from build123d import *

# Parameters (mm, degrees)
PAD_DEPTH       = 10
SKETCH001_R     = 17
POCKET_DEPTH    = 8
FILLET_R        = 2
FILLET001_R     = 2
SKETCH002_R     = 3
POCKET001_DEPTH = 5
FILLET002_R     = 2
FILLET003_R     = 2
SKETCH003_R     = 0.5
POCKET002_DEPTH = 5


with BuildPart() as part:
    # Sketch → Pad (new body)
    with BuildSketch(Plane.XY):
        with BuildLine():
            ThreePointArc((29.142732, 7.120476), (26.750427, 13.579935), (22.947847, 19.323465))
            Line((22.947847, 19.323465), (34.497449, 29.048923))
            ThreePointArc((34.497449, 29.048923), (0.205805, 45.098466), (-34.230891, 29.362562))
            Line((-22.770532, 19.532099), (-34.230891, 29.362562))
            ThreePointArc((-22.770532, 19.532099), (-26.452647, 14.151236), (-28.885266, 8.101937))
            Line((-28.885266, 8.101937), (-43.374809, 11.984403))
            ThreePointArc((-43.374809, 11.984403), (-43.973621, 9.556182), (-44.436607, 7.098445))
            Line((-44.436607, 7.098445), (-11.603749, -16.289659))
            ThreePointArc((-11.603749, -16.289659), (0.53379, -19.992875), (12.456435, -15.647276))
            Line((43.994501, 9.459593), (12.456435, -15.647276))
            ThreePointArc((43.994501, 9.459593), (43.401023, 11.889122), (42.673487, 14.281929))
            Line((29.142732, 7.120476), (42.673487, 14.281929))
        make_face()
    extrude(amount=PAD_DEPTH)

    # Sketch001 → Pocket (cut)
    with BuildSketch(Plane.XY.offset(10)):
        Circle(SKETCH001_R)
    extrude(amount=-POCKET_DEPTH, mode=Mode.SUBTRACT)

    # Fillet
    fillet_edges = [part.edges().sort_by_distance(p)[0] for p in [
        (-34.230891, 29.362562, 5),
    ]]
    fillet(fillet_edges, radius=FILLET_R)

    # Fillet001
    fillet001_edges = [part.edges().sort_by_distance(p)[0] for p in [
        (34.497449, 29.048923, 5),
    ]]
    fillet(fillet001_edges, radius=FILLET001_R)

    # Sketch002 → Pocket001 (cut)
    with BuildSketch(Plane.XY.offset(2)):
        Circle(SKETCH002_R)
    extrude(amount=-POCKET001_DEPTH, mode=Mode.SUBTRACT)

    # Fillet002
    fillet002_edges = [part.edges().sort_by_distance(p)[0] for p in [
        (-17, 0, 10),
    ]]
    fillet(fillet002_edges, radius=FILLET002_R)

    # Fillet003
    fillet003_edges = [part.edges().sort_by_distance(p)[0] for p in [
        (0.205805, 45.098466, 10),
    ]]
    fillet(fillet003_edges, radius=FILLET003_R)

    # Sketch003 → Pocket002 (cut)
    with BuildSketch(Plane.XY.offset(2)):
        with Locations((7.5, 3)):
            Circle(SKETCH003_R)
        with Locations((-7.5, -3)):
            Circle(SKETCH003_R)
    extrude(amount=-POCKET002_DEPTH, mode=Mode.SUBTRACT)


solid = part.part
Input: part model. Units: mm. Frame: model coordinates. A direction names the side the tool comes from. Coordinates: 2 decimals unless noted, no trailing zeros. Order: outer loops, then holes, each group sorted by start corner. A loop starts at its lowest first (then second) coordinate and runs counter-clockwise, first axis right, second up. Notation, with made-up numbers: M 28,17.5 L 36,17.5 A27 cw 36,53.5 Z; hole C 0.5,16.5 d2. An arc over 180 degrees is marked long. Answer in a Markdown table with one row per item.
(1) Section query B-B, the plane z = 6. Output: boundary loops of the cut face in (x, y).
Numbers:
| item | result |
|---|---|
| outline | M -44.44,7.1 L -11.6,-16.29 A20 ccw 12.46,-15.65 L 43.99,9.46 A45 ccw 42.67,14.28 L 29.14,7.12 A30 ccw 22.95,19.32 L 32.93,27.73 A2 ccw 33.11,30.62 A45.1 ccw -32.83,30.92 A2 ccw -32.68,28.03 L -22.77,19.53 A30 ccw -28.89,8.1 L -43.37,11.98 A45 ccw Z; hole C 0,0 d34 |
(2) Section query A-A, the plane y = 0. Output: boundary loops of the cut face in (x, z).
Numbers:
| item | result |
|---|---|
| outline | M -34.47,0 L -3,0 L -3,2 L -17,2 L -17,8 A2 ccw -19,10 L -34.47,10 Z; M 3,0 L 32.11,0 L 32.11,10 L 19,10 A2 ccw 17,8 L 17,2 L 3,2 Z |
(3) Material intervals for line 1 (Y direction, x = 0, z = 6.3); line 2 (Z direction, x = 10, y = -8); line 3 (X direction, y = -1.5, z = 4.5), sorted ascending. Write a range as [from, to].
Numbers:
| item | result |
|---|---|
| line 1 | y = [-20, -17], [17, 45.1] |
| line 2 | z = [0, 2] |
| line 3 | x = [-32.37, -16.93], [16.93, 30.23] |
(4) Access query for faces 4 (the flat face through (4, 0, 2)), 5 (the cylindrical face through (27.597, 24.025, 9.43)), 6 (the cylindrical face through (-27.24, 24.16, 9.43)), 7 (the flat face through (27.87, 23.47, 3.94)), 8 (the flat face through (-36.029, 10.016, 4.93)). Directions: +Z, -Z, +X, -X, +Y, -Y. A direction counts if a zero-diameter tool reaches every point of the face in a straight line with its end or side. Return the directions, or none.
Numbers:
| item | result |
|---|---|
| face 4 | +Z |
| face 5 | +Z, +X |
| face 6 | +Z, -X |
| face 7 | +Z, -Z, +X |
| face 8 | +Z, -Z |
(5) Contact query for flat-ended pins moving along their axis: pin 1 Ø1 at (x, z) = (-28, 5) entering from +Y; pin 2 Ø3 at (y, z) = (10, 8) entering from -X; pin 3 Ø6 at (x, z) = (29.5, 3.5) entering from -Y; pin 4 Ø3.5 at (x, y) = (0, 0) entering from +Z. Output: stop coordinate, or through.
Numbers:
| item | result |
|---|---|
| pin 1 | stops at y = 35.74 |
| pin 2 | stops at x = -44.19 |
| pin 3 | stops at y = -4.47 |
| pin 4 | passes through |
(6) Draft query along X for faces 1 (the cylindrical face through (-33.374, 29.465, 4.056)), 2 (the flat face through (35.81, 10.65, 4.93)), 3 (the cylindrical face through (43.4, 11.9, 4.9)). Return one class per face: pulls with the +X half, pulls with the -X half, needs draft (parallel to the pull), parting line crosses it, or undercut.
Numbers:
| item | result |
|---|---|
| face 1 | pulls with the -X half |
| face 2 | undercut |
| face 3 | pulls with the +X half |
